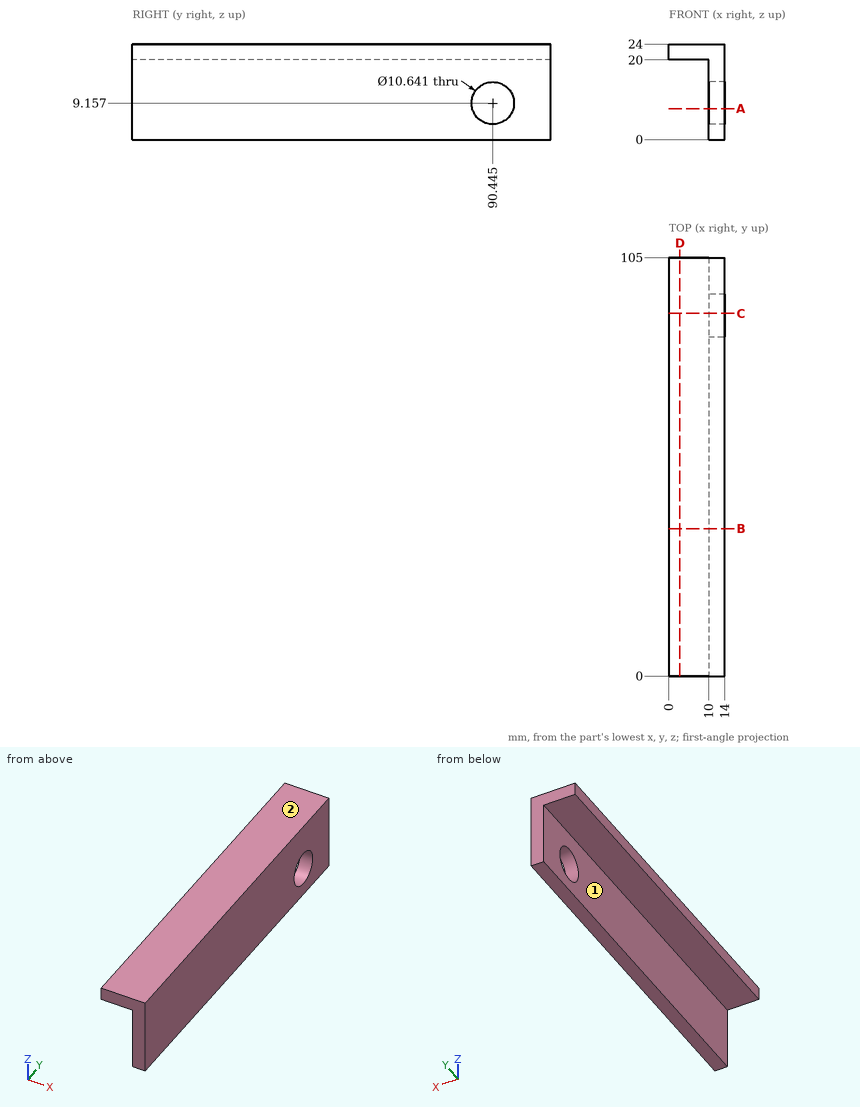
Job drawing, mm, ordinate dimensions from the low corner. One solid piece. A direction names the side the tool comes from. Coordinates: 2 decimals unless noted, no trailing zeros. Loops run counter-clockwise (first coordinate to the right, second up) from the corner with the lowest first, then second, coordinate; pieces in that order, holes last. Notation, with made-up numbers: (40.25, -24.5) - (50.25, -24.5) arc R27 ccw to (50.25, 8.5) - close; hole circle Ø6 at (84, 11). An arc over 180 degrees is marked (long way). Answer as a JSON object with one key per item and string values. Group by question number.
(1) Flat gauge pins, fed straight in: pin 1 (1 mm diameter, centred on x = 10.5, z = 17.5, fed in from -Y); pin 2 (3 mm diameter, centred on x = 6.5, y = 60.5, fed in from -Z); pin 3 (1.5 mm diameter, centred on x = 3.5, z = 18, fed in from +Y). Where does each tip first touch, or does it go through?
(2) Cut at C-C (y = 91). Give the cut face in (x, z) (1 decimal).
(3) Cut at B-B (y = 37). Give the cut face in (x, z).
(4) Cut at A-A (z = 7.75). Give the cut face in (x, y).
(5) Tool access for the marked faces 1 and 2: list every direction of +Z, -Z, +X, -X, +Y, -Y with a clear straight run to the whole face (end or side of a thin tool).
(6) Cut at D-D (x = 2.75). Give the cut face in (y, z).
(7) Probe line 1 along Z through (x, y) = (1.25, 80); line 2 along X through (y, z) = (13, 3.75); line 3 along Y through (x, z) = (12, 10). List the from-to ranges inside material, lowest first.
Geometry says:
{
 "1": {"pin 1": "stops at y = 0", "pin 2": "stops at z = 20", "pin 3": "passes through"},
 "2": {"outline": "(0, 20) - (10, 20) - (10, 14.4) - (14, 14.4) - (14, 24) - (0, 24) - close; (10, 0) - (14, 0) - (14, 3.9) - (10, 3.9) - close"},
 "3": {"outline": "(0, 20) - (10, 20) - (10, 0) - (14, 0) - (14, 24) - (0, 24) - close"},
 "4": {"outline": "(10, 0) - (14, 0) - (14, 85.31) - (10, 85.31) - close; (10, 95.58) - (14, 95.58) - (14, 105) - (10, 105) - close"},
 "5": {"face 1": "-Z, -X, +Y, -Y", "face 2": "+Z, +X, -X, +Y, -Y"},
 "6": {"outline": "(0, 20) - (105, 20) - (105, 24) - (0, 24) - close"},
 "7": {"line 1": "z = 20 to 24", "line 2": "x = 10 to 14", "line 3": "y = 0 to 85.19, 95.7 to 105"}
}
